Design review of the part built by this model. Coordinates are the model's own, in mm. A direction names the side the tool comes from. Give positions to 0.01 mm unless a question says otherwise; leave off trailing zeros. Write each loop counter-clockwise with the first axis right and the second up, starting at its lowest first coordinate (ties: lowest second). Pieces come first, ordered by that corner, then holes. Notation, with made-up numbers: (56, 57) -> (63, 57) arc R17 ccw to (63, 86) -> close; hole circle Ø11 at (33.25, 58). An arc over 180 degrees is marked (long way). Answer as a JSON object with one key per item and string values.
Autodesk Inventor part; units mm, degrees
ref_plane "YZ Plane" through (0, 0, 0) normal (1, 0, 0) x (0, 1, 0)
ref_plane "XZ Plane" through (0, 0, 0) normal (0, 1, 0) x (-1, 0, 0)
ref_plane "XY Plane" through (0, 0, 0) normal (0, 0, 1) x (1, 0, 0)
sketch "Sketch1" plane through (0, 0, 0) normal (0, 0, 1) x (1, 0, 0)
  line L0 (0, 0) -> (152.4, 0)
  line L1 (152.4, 25.4) -> (152.4, 127)
  line L2 (152.4, 152.4) -> (0, 152.4)
  line L3 (0, 127) -> (0, 25.4)
  circle A0 centre (25.4, 127) radius 1.5875
  circle A1 centre (50.8, 127) radius 1.5875
  circle A2 centre (76.2, 127) radius 1.5875
  circle A3 centre (101.6, 127) radius 1.5875
  circle A4 centre (127, 127) radius 1.5875
  circle A5 centre (25.4, 25.4) radius 1.5875
  circle A6 centre (50.8, 25.4) radius 1.5875
  circle A7 centre (76.2, 25.4) radius 1.5875
  circle A8 centre (101.6, 25.4) radius 1.5875
  circle A9 centre (127, 25.4) radius 1.5875
  line L4 (41.275, 36.6265) -> (15.875, 36.6265)
  line L5 (15.875, 36.6265) -> (28.575, 58.6235)
  line L6 (28.575, 58.6235) -> (41.275, 36.6265)
  line L7 (60.325, 58.6235) -> (47.625, 36.6265)
  line L8 (47.625, 36.6265) -> (34.925, 58.6235)
  line L9 (34.925, 58.6235) -> (60.325, 58.6235)
  line L10 (98.425, 58.6235) -> (85.725, 36.6265)
  line L11 (73.025, 58.6235) -> (98.425, 58.6235)
  line L12 (85.725, 36.6265) -> (73.025, 58.6235)
  line L13 (66.675, 58.6235) -> (79.375, 36.6265)
  line L14 (53.975, 36.6265) -> (66.675, 58.6235)
  line L15 (79.375, 36.6265) -> (53.975, 36.6265)
  line L16 (136.525, 58.6235) -> (123.825, 36.6265)
  line L17 (111.125, 58.6235) -> (136.525, 58.6235)
  line L18 (123.825, 36.6265) -> (111.125, 58.6235)
  line L19 (104.775, 58.6235) -> (117.475, 36.6265)
  line L20 (92.075, 36.6265) -> (104.775, 58.6235)
  line L21 (117.475, 36.6265) -> (92.075, 36.6265)
  line L22 (0, 36.6265) -> (15.875, 36.6265)
  line L23 (136.525, 58.6235) -> (152.4, 58.6235)
  line L24 (104.775, 87.1985) -> (117.475, 65.2015)
  line L25 (123.825, 65.2015) -> (111.125, 87.1985)
  line L26 (136.525, 87.1985) -> (123.825, 65.2015)
  line L27 (111.125, 87.1985) -> (136.525, 87.1985)
  line L28 (117.475, 65.2015) -> (92.075, 65.2015)
  line L29 (41.275, 65.2015) -> (15.875, 65.2015)
  line L30 (15.875, 65.2015) -> (28.575, 87.1985)
  line L31 (28.575, 87.1985) -> (41.275, 65.2015)
  line L32 (60.325, 87.1985) -> (47.625, 65.2015)
  line L33 (47.625, 65.2015) -> (34.925, 87.1985)
  line L34 (34.925, 87.1985) -> (60.325, 87.1985)
  line L35 (92.075, 65.2015) -> (104.775, 87.1985)
  line L36 (73.025, 87.1985) -> (98.425, 87.1985)
  line L37 (85.725, 65.2015) -> (73.025, 87.1985)
  line L38 (66.675, 87.1985) -> (79.375, 65.2015)
  line L39 (53.975, 65.2015) -> (66.675, 87.1985)
  line L40 (79.375, 65.2015) -> (53.975, 65.2015)
  line L41 (98.425, 87.1985) -> (85.725, 65.2015)
  line L42 (104.775, 115.7735) -> (117.475, 93.7765)
  line L43 (123.825, 93.7765) -> (111.125, 115.7735)
  line L44 (136.525, 115.7735) -> (123.825, 93.7765)
  line L45 (111.125, 115.7735) -> (136.525, 115.7735)
  line L46 (117.475, 93.7765) -> (92.075, 93.7765)
  line L47 (41.275, 93.7765) -> (15.875, 93.7765)
  line L48 (15.875, 93.7765) -> (28.575, 115.7735)
  line L49 (28.575, 115.7735) -> (41.275, 93.7765)
  line L50 (60.325, 115.7735) -> (47.625, 93.7765)
  line L51 (47.625, 93.7765) -> (34.925, 115.7735)
  line L52 (34.925, 115.7735) -> (60.325, 115.7735)
  line L53 (92.075, 93.7765) -> (104.775, 115.7735)
  line L54 (73.025, 115.7735) -> (98.425, 115.7735)
  line L55 (85.725, 93.7765) -> (73.025, 115.7735)
  line L56 (66.675, 115.7735) -> (79.375, 93.7765)
  line L57 (53.975, 93.7765) -> (66.675, 115.7735)
  line L58 (79.375, 93.7765) -> (53.975, 93.7765)
  line L59 (98.425, 115.7735) -> (85.725, 93.7765)
  line L60 (15.875, 36.6265) -> (15.875, 0)
  line L61 (28.575, 115.7735) -> (28.575, 152.4)
  line L62 (12.7, 12.7) -> (139.7, 12.7)
  line L63 (12.7, 139.7) -> (139.7, 139.7)
  arc A10 (0, 25.4) -> (12.7, 12.7) centre (12.7, 25.4) ccw
  arc A11 (139.7, 12.7) -> (152.4, 25.4) centre (139.7, 25.4) ccw
  arc A12 (152.4, 127) -> (139.7, 139.7) centre (139.7, 127) ccw
  arc A13 (12.7, 139.7) -> (0, 127) centre (12.7, 127) ccw
  point P0 (28.575, 43.9588)
  point P1 (28.575, 36.6265)
  point P2 (47.625, 51.2912)
  point P3 (85.725, 51.2912)
  point P4 (66.675, 43.9588)
  point P5 (66.675, 36.6265)
  point P6 (123.825, 51.2912)
  point P7 (104.775, 43.9588)
  point P8 (104.775, 36.6265)
  point P9 (123.825, 79.8662)
  point P10 (104.775, 65.2015)
  point P11 (28.575, 72.5338)
  point P12 (28.575, 65.2015)
  point P13 (47.625, 79.8662)
  point P14 (104.775, 72.5338)
  point P15 (85.725, 79.8662)
  point P16 (66.675, 72.5338)
  point P17 (66.675, 65.2015)
  point P18 (123.825, 108.4412)
  point P19 (104.775, 93.7765)
  point P20 (28.575, 101.1088)
  point P21 (28.575, 93.7765)
  point P22 (47.625, 108.4412)
  point P23 (104.775, 101.1088)
  point P24 (85.725, 108.4412)
  point P25 (66.675, 101.1088)
  point P26 (66.675, 93.7765)
  dimension "d0" = 152.4
  dimension "d1" = 152.4
  dimension "d2" = 3.175
  dimension "d3" = 25.4
  dimension "d4" = 25.4
  dimension "d7" = 25.4
  dimension "d12" = 3.175
  dimension "d13" = 25.4
  dimension "d14" = 25.4
  dimension "d17" = 25.4
  dimension "d22" = 25.4
  dimension "d23" = 25.4
  dimension "d24" = 0
  dimension "d25" = 6.35
  dimension "d29" = 38.1
  dimension "d37" = 28.575
  dimension "d42" = 12.7
  dimension "d43" = 12.7
  dimension "d44" = 12.7
extrude "Extrusion1" add sketch "Sketch1" along normal blind 3.175
properties part number "Low Frame to Mid Frame bracket"
(1) Clearance check with a flat-ended pin moving along its axis: pin 1 (3 mm diameter, centred on x = 127, y = 25.4, fed in from -Z). State where the tip first meets the part, or that it passes through.
Here are the results:
{"pin 1": "passes through"}
(2) For faces 1 (the flat face through (29, 93.776, 2)), 2 (the cylindrical face through (148.58, 136.08, 1.57)), list the 3-axis set-ups (+Z, -Z, +X, -X, +Y, -Y) from which the entire face can be reached by the end or side of a thin tool; tool diameter is ignored.
Here are the results:
{"face 1": "+Z, -Z", "face 2": "+Z, -Z, +X, +Y"}
(3) For line 1 along X through (y, z) = (127, 0.9); line 2 along Y through (x, z) = (66, 2.2); line 3 along Y through (x, z) = (25.4, 0.9), list the stretches that pass through material, from the lowest coordinate up.
Here are the results:
{"line 1": "x = 0 to 23.81, 26.99 to 49.21, 52.39 to 74.61, 77.79 to 100.01, 103.19 to 125.41, 128.59 to 152.4", "line 2": "y = 12.7 to 36.63, 57.45 to 65.2, 86.03 to 93.78, 114.6 to 139.7", "line 3": "y = 12.7 to 23.81, 26.99 to 36.63, 53.12 to 65.2, 81.7 to 93.78, 110.27 to 125.41, 128.59 to 139.7"}
(4) We need section B-B, the plane y = 46.5. State the section outline as (x, z) points (3 decimals), then the cut area to 3 significant figures.
Here are the results:
{"outline": "(0, 0) -> (21.575, 0) -> (21.575, 3.175) -> (0, 3.175) -> close; (35.575, 0) -> (41.925, 0) -> (41.925, 3.175) -> (35.575, 3.175) -> close; (53.325, 0) -> (59.675, 0) -> (59.675, 3.175) -> (53.325, 3.175) -> close; (73.675, 0) -> (80.025, 0) -> (80.025, 3.175) -> (73.675, 3.175) -> close; (91.425, 0) -> (97.775, 0) -> (97.775, 3.175) -> (91.425, 3.175) -> close; (111.775, 0) -> (118.125, 0) -> (118.125, 3.175) -> (111.775, 3.175) -> close; (129.525, 0) -> (152.4, 0) -> (152.4, 3.175) -> (129.525, 3.175) -> close", "area": "242 mm²"}
(5) We need section A-A, the plane x = 134. State the section outline as (y, z) points (1 decimal), then the cut area to 3 significant figures.
Here are the results:
{"outline": "(12.7, 0) -> (54.3, 0) -> (54.3, 3.2) -> (12.7, 3.2) -> close; (58.6, 0) -> (82.8, 0) -> (82.8, 3.2) -> (58.6, 3.2) -> close; (87.2, 0) -> (111.4, 0) -> (111.4, 3.2) -> (87.2, 3.2) -> close; (115.8, 0) -> (139.7, 0) -> (139.7, 3.2) -> (115.8, 3.2) -> close", "area": "362 mm²"}
(6) The part is to be moulded in two halves that separate along X. For faces 3 (the flat face through (0, 77, 2)), 4 (the cylindrical face through (148.78, 16.52, 1.57)), 5 (the flat face through (41.364, 47.471, 1.565)), say which applies: +X half, -X half, draft (parallel to the pull), parting line (faces both ways), or undercut.
Here are the results:
{"face 3": "-X half", "face 4": "+X half", "face 5": "undercut"}
(7) We need section C-C, the plane x = 70. State the section outline as (y, z) points (1 decimal), then the cut area to 3 significant figures.
Here are the results:
{"outline": "(12.7, 0) -> (36.6, 0) -> (36.6, 3.2) -> (12.7, 3.2) -> close; (52.9, 0) -> (65.2, 0) -> (65.2, 3.2) -> (52.9, 3.2) -> close; (81.4, 0) -> (93.8, 0) -> (93.8, 3.2) -> (81.4, 3.2) -> close; (110, 0) -> (139.7, 0) -> (139.7, 3.2) -> (110, 3.2) -> close", "area": "249 mm²"}
(8) We need section D-D, the plane z = 2.55. Give the number of separate pieces and of enclosed holes in the cut face, then the cut area to 3 significant figures.
Here are the results:
{"separate pieces": "1", "enclosed holes": "28", "area": "14,100 mm²"}
